Source: CAD feature listing. Evaluate the final solid. Frame: model axes, mm. Give positions to 0.01 mm unless a question says otherwise; leave off trailing zeros. Loops run counter-clockwise (first coordinate to the right, second up) from the corner with the lowest first, then second, coordinate; pieces in that order, holes last. Notation, with made-up numbers: (10, -3.75) - (63, -3.75) arc R26 ccw to (63, 14.25) - close; hole circle Ø5 at (27.5, -15). An arc over 180 degrees is marked (long way). Write each question's results on one line, items separated by ' | '. Start each with the question number.
(1) Cut plane B-B on z = 22. Return the cut outline in (x, y), then the cut area to 3 significant figures.
(2) Cut plane A-A on y = 35. Return the cut outline in (x, z), then the cut area to 3 significant figures.
(3) Contact query for flat-ended pins moving along their axis: pin 1 (6 mm diameter, centred on x = 14, y = 23, fed in from -Z); pin 2 (3 mm diameter, centred on y = 17.65, z = 210, fed in from -X); pin 3 (2 mm diameter, centred on x = 10, z = 250, fed in from -Y). Output: stop coordinate, or through.
(4) Material intervals for line 1 along X through (y, z) = (0.4, 170); line 2 along Y through (x, z) = (3, 111.5); line 3 along X through (y, z) = (24.5, 245), sorted ascending. Write a range as [from, to].
from build123d import *

# Parameters (mm, degrees)
SKETCH_1_W          = 20
SKETCH_1_H          = 40
SKETCH_1_W_2        = 16
SKETCH_1_H_2        = 36
EXTRUDE_1_DEPTH     = 315
SKETCH_2_R          = 2
CUT_EXTRUDE_1_DEPTH = 319.158765399
SKETCH_3_R          = 1.75
CUT_EXTRUDE_2_DEPTH = 2
SKETCH_4_R          = 1.75
CUT_EXTRUDE_3_DEPTH = 2


with BuildPart() as part:
    # 草图1 → 凸台-拉伸1 (new body)
    with BuildSketch(Plane.XY):
        with Locations((10, 20)):
            Rectangle(SKETCH_1_W, SKETCH_1_H)
        with Locations((10, 20)):
            Rectangle(SKETCH_1_W_2, SKETCH_1_H_2, mode=Mode.SUBTRACT)
    extrude(amount=EXTRUDE_1_DEPTH)

    # 草图2 → 切除-拉伸1 (cut, through all)
    with BuildSketch(Plane(origin=(20, 0, 0), x_dir=(0, 0, -1), z_dir=(1, 0, 0))):
        with Locations((-290, 30)):
            Circle(SKETCH_2_R)
        with Locations((-15, 10)):
            Circle(SKETCH_2_R)
    extrude(amount=-CUT_EXTRUDE_1_DEPTH, mode=Mode.SUBTRACT)

    # 草图3 → 切除-拉伸2 (cut)
    with BuildSketch(Plane.ZY):
        with Locations((10, 17.65)):
            Circle(SKETCH_3_R)
        with Locations((30, 17.65)):
            Circle(SKETCH_3_R)
        with Locations((50, 17.65)):
            Circle(SKETCH_3_R)
        with Locations((70, 17.65)):
            Circle(SKETCH_3_R)
        with Locations((90, 17.65)):
            Circle(SKETCH_3_R)
        with Locations((110, 17.65)):
            Circle(SKETCH_3_R)
        with Locations((130, 17.65)):
            Circle(SKETCH_3_R)
        with Locations((150, 17.65)):
            Circle(SKETCH_3_R)
        with Locations((170, 17.65)):
            Circle(SKETCH_3_R)
        with Locations((190, 17.65)):
            Circle(SKETCH_3_R)
        with Locations((210, 17.65)):
            Circle(SKETCH_3_R)
        with Locations((230, 17.65)):
            Circle(SKETCH_3_R)
        with Locations((250, 17.65)):
            Circle(SKETCH_3_R)
        with Locations((270, 17.65)):
            Circle(SKETCH_3_R)
    extrude(amount=-CUT_EXTRUDE_2_DEPTH, mode=Mode.SUBTRACT)

    # 草图4 → 切除-拉伸3 (cut)
    with BuildSketch(Plane(origin=(0, 0, 0), x_dir=(-1, 0, 0), z_dir=(0, -1, 0))):
        with Locations(Location((-10, -10, 0), (0, 0, 90))):
            Circle(SKETCH_4_R)
        with Locations(Location((-10, -30, 0), (0, 0, 90))):
            Circle(SKETCH_4_R)
        with Locations(Location((-10, -50, 0), (0, 0, 90))):
            Circle(SKETCH_4_R)
        with Locations(Location((-10, -70, 0), (0, 0, 90))):
            Circle(SKETCH_4_R)
        with Locations(Location((-10, -90, 0), (0, 0, 90))):
            Circle(SKETCH_4_R)
        with Locations(Location((-10, -110, 0), (0, 0, 90))):
            Circle(SKETCH_4_R)
        with Locations(Location((-10, -130, 0), (0, 0, 90))):
            Circle(SKETCH_4_R)
        with Locations(Location((-10, -150, 0), (0, 0, 90))):
            Circle(SKETCH_4_R)
        with Locations(Location((-10, -170, 0), (0, 0, 90))):
            Circle(SKETCH_4_R)
        with Locations(Location((-10, -190, 0), (0, 0, 90))):
            Circle(SKETCH_4_R)
        with Locations(Location((-10, -210, 0), (0, 0, 90))):
            Circle(SKETCH_4_R)
        with Locations(Location((-10, -230, 0), (0, 0, 90))):
            Circle(SKETCH_4_R)
        with Locations(Location((-10, -250, 0), (0, 0, 90))):
            Circle(SKETCH_4_R)
        with Locations(Location((-10, -270, 0), (0, 0, 90))):
            Circle(SKETCH_4_R)
    extrude(amount=-CUT_EXTRUDE_3_DEPTH, mode=Mode.SUBTRACT)


solid = part.part
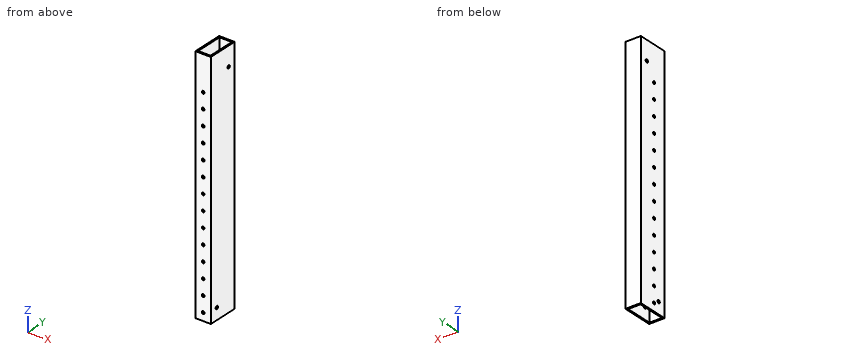
Ans:
1) outline: (0, 0) - (20, 0) - (20, 40) - (0, 40) - close; hole (2, 2) - (18, 2) - (18, 38) - (2, 38) - close | area: 224 mm^2
2) outline: (0, 0) - (2, 0) - (2, 315) - (0, 315) - close; (18, 0) - (20, 0) - (20, 315) - (18, 315) - close | area: 1,260 mm^2
3) pin 1: through | pin 2: x = 18 | pin 3: y = 38
4) line 1: [0, 8.25], [11.75, 20] | line 2: [0, 2], [38, 40] | line 3: [0, 2], [18, 20]
